Input: dimensioned drawing with shaded views. Units: mm. Origin: part minimum x, y, z. Give positions to 0.01 mm unless a question says otherwise; leave off trailing zeros. Write each loop counter-clockwise with the first axis right and the second up, starting at its lowest first coordinate (ties: lowest second). Pieces come first, ordered by that corner, then holes.
Q1. Pin query (flat end, axial travel): pin 1 Ø7 at (x, y) = (115, 15) entering from +Z; pin 2 Ø10.5 at (x, y) = (15, 15) entering from -Z. Return the tip coordinate at first contact, or that it passes through.
Q2. Section B-B (z = 1.6). Return the cut outline in (x, y).
Q3. Section C-C (x = 15). Return the cut outline in (y, z).
Q4. Section A-A (y = 15). Return the cut outline in (x, z), plus the area to 3 significant figures.
Q5. Line query: line 1 (X direction, y = 44.5, z = 0.2); line 2 (X direction, y = 13.5, z = 1.6) (1 decimal); line 3 (X direction, y = 14, z = 1.85) (1 decimal). Output: solid intervals per line, ascending.
Q6. Section D-D (x = 69.5). Return the cut outline in (y, z).
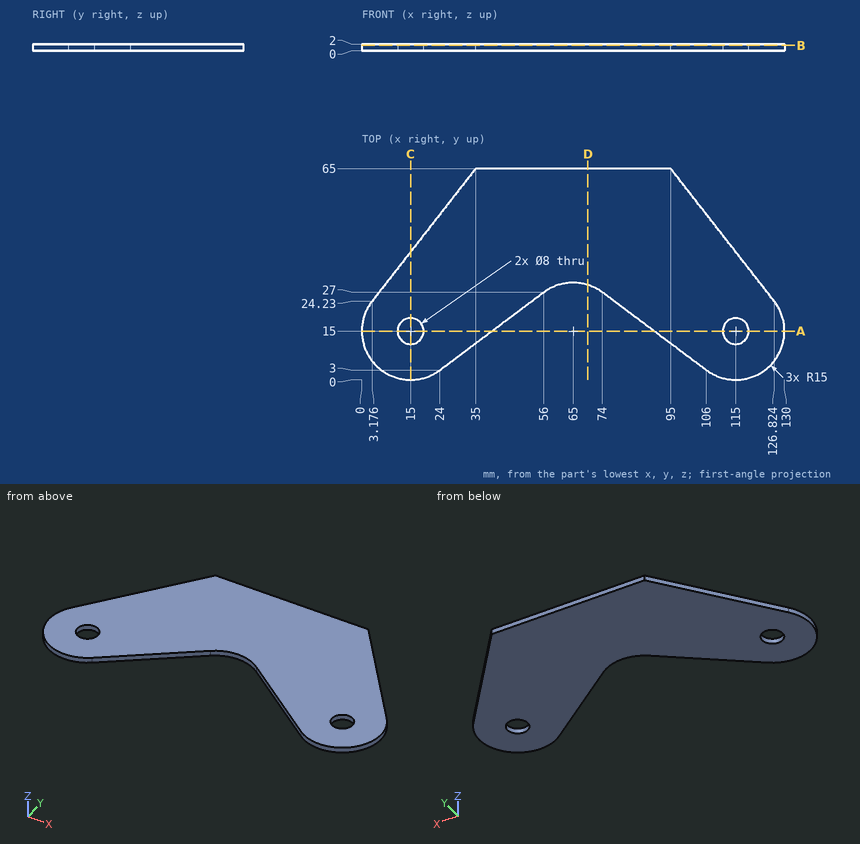
Computed:
1. pin 1: passes through
1. pin 2: stops at z = 0
2. outline: (3.18, 24.23) arc R15 ccw to (24, 3) - (56, 27) arc R15 cw to (74, 27) - (106, 3) arc R15 ccw to (126.82, 24.23) - (95, 65) - (35, 65) - close; hole circle Ø8 at (15, 15); hole circle Ø8 at (115, 15)
3. outline: (0, 0) - (11, 0) - (11, 2) - (0, 2) - close; (19, 0) - (39.38, 0) - (39.38, 2) - (19, 2) - close
4. outline: (0, 0) - (11, 0) - (11, 2) - (0, 2) - close; (19, 0) - (40, 0) - (40, 2) - (19, 2) - close; (90, 0) - (111, 0) - (111, 2) - (90, 2) - close; (119, 0) - (130, 0) - (130, 2) - (119, 2) - close
4. area: 128 mm2
5. line 1: x = 19 to 111
5. line 2: x = 0.1 to 11.3, 18.7 to 38, 92 to 111.3, 118.7 to 129.9
5. line 3: x = 0 to 11.1, 18.9 to 38.7, 91.3 to 111.1, 118.9 to 130
6. outline: (29.31, 0) - (65, 0) - (65, 2) - (29.31, 2) - close
